Geometry check sheet. Reference: the model listing, model coordinates, mm. A direction names the side the tool comes from. Give positions to 0.01 mm unless a question says otherwise; leave off trailing zeros. Order: outer loops, then holes, each group sorted by start corner. A loop starts at its lowest first (then second) coordinate and runs counter-clockwise, first axis right, second up.
```python
from build123d import *

# Parameters (mm, degrees)
F0_W     = 20
F0_H     = 20
F0_W_2   = 19.2
F0_H_2   = 19.2
F1_DEPTH = 75
F2_R     = 1.5
F3_DEPTH = 0.4
F5_DEPTH = 0.4
F7_DEPTH = 0.4


with BuildPart() as f1:
    # F0 (on Top) → F1 (new body)
    with BuildSketch(Plane.XY):
        Rectangle(F0_W, F0_H)
        Rectangle(F0_W_2, F0_H_2, mode=Mode.SUBTRACT)
    extrude(amount=F1_DEPTH)

    # F2 (on face) → F3 (cut, through all)
    with BuildSketch(Plane(origin=(0, 10, 0), x_dir=(-1, 0, 0), z_dir=(0, 1, 0))):
        with Locations((0, 62.5)):
            Circle(F2_R)
        with Locations((0, 52.5)):
            Circle(F2_R)
        with Locations((0, 42.5)):
            Circle(F2_R)
        with Locations((0, 32.5)):
            Circle(F2_R)
        with Locations((0, 22.5)):
            Circle(F2_R)
        with Locations((0, 12.5)):
            Circle(F2_R)
        with Locations((0, 72.5)):
            Circle(F2_R)
    extrude(amount=-F3_DEPTH, mode=Mode.SUBTRACT)

    # F4 (on face) → F5 (cut, through all)
    with BuildSketch(Plane.XZ.offset(10)):
        Polygon((2.886751, 10), (-2.886751, 10), (0, 5), align=None)
        Polygon((-2.886751, 20), (0, 15), (2.886751, 20), align=None)
        Polygon((-2.886751, 30), (0, 25), (2.886751, 30), align=None)
        Polygon((-2.886751, 40), (0, 35), (2.886751, 40), align=None)
        Polygon((-2.886751, 50), (0, 45), (2.886751, 50), align=None)
        Polygon((-2.886751, 60), (0, 55), (2.886751, 60), align=None)
        Polygon((-2.886751, 70), (0, 65), (2.886751, 70), align=None)
    extrude(amount=-F5_DEPTH, mode=Mode.SUBTRACT)

    # F6 (on face) → F7 (cut, through all)
    with BuildSketch(Plane(origin=(-10, 0, 0), x_dir=(0, -1, 0), z_dir=(-1, 0, 0))):
        with BuildLine():
            ThreePointArc((-1.792893, 10.707107), (-3.207107, 10.707107), (-3.207107, 9.292893))
            Line((-3.207107, 9.292893), (1.792893, 4.292893))
            ThreePointArc((1.792893, 4.292893), (3.207107, 4.292893), (3.207107, 5.707107))
            Line((3.207107, 5.707107), (-1.792893, 10.707107))
        make_face()
        with BuildLine():
            ThreePointArc((-1.792893, 20.707107), (-3.207107, 20.707107), (-3.207107, 19.292893))
            Line((-3.207107, 19.292893), (1.792893, 14.292893))
            ThreePointArc((1.792893, 14.292893), (3.207107, 14.292893), (3.207107, 15.707107))
            Line((3.207107, 15.707107), (-1.792893, 20.707107))
        make_face()
        with BuildLine():
            ThreePointArc((-1.792893, 30.707107), (-3.207107, 30.707107), (-3.207107, 29.292893))
            Line((-3.207107, 29.292893), (1.792893, 24.292893))
            ThreePointArc((1.792893, 24.292893), (3.207107, 24.292893), (3.207107, 25.707107))
            Line((3.207107, 25.707107), (-1.792893, 30.707107))
        make_face()
        with BuildLine():
            ThreePointArc((-1.792893, 40.707107), (-3.207107, 40.707107), (-3.207107, 39.292893))
            Line((-3.207107, 39.292893), (1.792893, 34.292893))
            ThreePointArc((1.792893, 34.292893), (3.207107, 34.292893), (3.207107, 35.707107))
            Line((3.207107, 35.707107), (-1.792893, 40.707107))
        make_face()
        with BuildLine():
            ThreePointArc((-1.792893, 50.707107), (-3.207107, 50.707107), (-3.207107, 49.292893))
            Line((-3.207107, 49.292893), (1.792893, 44.292893))
            ThreePointArc((1.792893, 44.292893), (3.207107, 44.292893), (3.207107, 45.707107))
            Line((3.207107, 45.707107), (-1.792893, 50.707107))
        make_face()
        with BuildLine():
            ThreePointArc((-1.792893, 60.707107), (-3.207107, 60.707107), (-3.207107, 59.292893))
            Line((-3.207107, 59.292893), (1.792893, 54.292893))
            ThreePointArc((1.792893, 54.292893), (3.207107, 54.292893), (3.207107, 55.707107))
            Line((3.207107, 55.707107), (-1.792893, 60.707107))
        make_face()
        with BuildLine():
            ThreePointArc((-1.792893, 70.707107), (-3.207107, 70.707107), (-3.207107, 69.292893))
            Line((-3.207107, 69.292893), (1.792893, 64.292893))
            ThreePointArc((1.792893, 64.292893), (3.207107, 64.292893), (3.207107, 65.707107))
            Line((3.207107, 65.707107), (-1.792893, 70.707107))
        make_face()
    extrude(amount=-F7_DEPTH, mode=Mode.SUBTRACT)


solid = f1.part
```
Q1. Gauge pin test, flat ends, axial feed: P1, Ø1.8, axis at x = 0, z = 22.5, coming from the +Y side; P2, Ø8, axis at x = 4, y = -0.5, coming from the +Z side. Record the tip position at first contact, or that the pin passes through.
Q2. Access from +Z, -Z, +X, -X, +Y, -Y to the whole of each face (thin tool, end or side, straight path). Record for faces 3 (the face through (-1.464, -9.803, 7.535)), 4 (the face through (0.325, 9.803, 31.036)), 5 (the face through (-9.803, 0.742, 6.828)), 6 (the face through (-2, -9.6, 37)), 7 (the face through (10, 0, 37)).
Q3. Cross-section at A-A, the plane x = 5.75. Record the boundary of the cut face in (y, z), and give its area (3 significant figures).
Q4. Cross-section at C-C, the plane z = 12.5. Record the boundary of the cut face in (x, y), and give its area (3 significant figures).
Q5. Thickness scan on L1, parallel to X at y = 4, z = 36; L2, parallel to X at y = 9.8, z = 72.5. Record the ranges inside material, lowest first.
Q6. Cross-section at D-D, the plane y = 2.5. Give the number of separate pieces and of enclosed holes in the cut face, and give its area (3 significant figures).
Q7. Release check for a two-part mould opening along Y. For faces 1 (the face through (1.42, -9.8, 47.46)), 2 (the face through (-9.803, 3.191, 40.722)) record: pulls with the +Y half, pulls with the -Y half, needs draft (parallel to the pull), parting line crosses it, or undercut.
Answers follow:
1. P1: stops at y = -9.6
1. P2: passes through
2. face 3: -Y
2. face 4: +Y
2. face 5: -X
2. face 6: +Z, -Z
2. face 7: +Z, -Z, +X, +Y, -Y
3. outline: (-10, 0) - (-9.6, 0) - (-9.6, 75) - (-10, 75) - close; (9.6, 0) - (10, 0) - (10, 75) - (9.6, 75) - close
3. area: 60.0 mm2
4. outline: (-10, -10) - (10, -10) - (10, 10) - (1.5, 10) - (1.5, 9.6) - (9.6, 9.6) - (9.6, -9.6) - (-9.6, -9.6) - (-9.6, 9.6) - (-1.5, 9.6) - (-1.5, 10) - (-10, 10) - close
4. area: 30.2 mm2
5. L1: x = -10 to -9.6, 9.6 to 10
5. L2: x = -10 to -1.5, 1.5 to 10
6. separate pieces: 9
6. enclosed holes: 0
6. area: 53.2 mm2
7. face 1: needs draft
7. face 2: undercut
